Input: part model. Units: mm. Frame: model coordinates. Coordinates: 2 decimals unless noted, no trailing zeros. Write each loop counter-clockwise with the first axis right and the second up, starting at its lowest first coordinate (ties: lowest second). Pieces come first, ordered by that corner, then holes. Notation, with made-up numbers: M -18,60.5 L 35,60.5 A26 cw 35,81.5 Z; hole C 10.25,17.25 d9. An arc over 180 degrees is marked long. Answer as a JSON object with one key per item and string values. Group by question number.
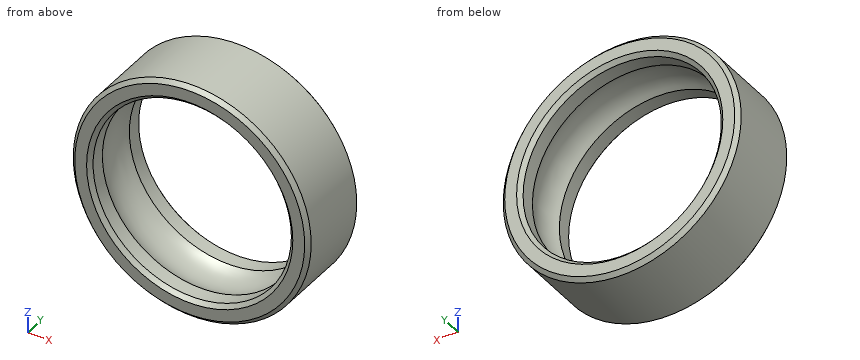
from build123d import *

# Parameters (mm, degrees)
SKETCH1_R           = 6
SKETCH1_R_2         = 5
BOSS_EXTRUDE1_DEPTH = 2
CHAMFER1_SIZE       = 0.2
SKETCH2_R           = 1.8


with BuildPart() as part:
    # Sketch1 → Boss-Extrude1 (new body, symmetric)
    with BuildSketch(Plane(origin=(0, 0, 0), x_dir=(1, 0, 0), z_dir=(0, 1, 0))):
        Circle(SKETCH1_R)
        Circle(SKETCH1_R_2, mode=Mode.SUBTRACT)
    extrude(amount=BOSS_EXTRUDE1_DEPTH, both=True)

    # Chamfer1
    chamfer1_edges = [part.edges().sort_by_distance(p)[0] for p in [
        (-6, -2, 0),
        (-6, 2, 0),
        (-5, -2, 0),
        (-5, 2, 0),
    ]]
    chamfer(chamfer1_edges, length=CHAMFER1_SIZE)

    # Cut-Sweep1: sweep along a path in Sketch3
    with BuildLine(Plane(origin=(0, 0, 0), x_dir=(1, 0, 0), z_dir=(0, 1, 0))) as cut_sweep1_path:
        CenterArc((0, 0), 3.542184236, 0, 360)
    # Sketch2 → Cut-Sweep1 (sweep, cut)
    with BuildSketch(Plane(origin=(0, 0, 0), x_dir=(0, 0, -1), z_dir=(1, 0, 0))):
        with Locations((-3.549093178, 0)):
            Circle(SKETCH2_R)
    sweep(path=cut_sweep1_path.line, mode=Mode.SUBTRACT)


solid = part.part
Q1. Section A-A, the plane x = 0. Return the cut outline in (y, z), and give its area (3 significant figures).
Q2. Line query: line 1 (X direction, y = 1.6, z = 0); line 2 (Z direction, x = -2, y = 0.75). Output: solid intervals per line, ascending. Write a range as from..to.
Q3. Pin query (flat end, axial travel): pin 1 Ø3 at (x, z) = (-0.5, -3.5) entering from -Y; pin 2 Ø1.5 at (y, z) = (-1.5, 1) entering from +X; pin 3 Ø1.5 at (x, z) = (3.5, -2.5) entering from -Y; pin 4 Ø3 at (x, z) = (-1.5, 2) entering from +Y. Return the tip coordinate at first contact, or that it passes through.
Q4. Section B-B, the plane z = 0. Return the cut outline in (x, y), and give its area (3 significant figures).
Q5. Section C-C, the plane y = -0.3. Return the cut outline in (x, z).
Q6. Section D-D, the plane y = 0.9. Return the cut outline in (x, z).
Filled in:
{
 "1": {"outline": "M -2,-5.8 L -1.8,-6 L 1.8,-6 L 2,-5.8 L 2,-5.2 L 1.8,-5 L 1.07,-5 A1.8 cw -1.07,-5 L -1.8,-5 L -2,-5.2 Z; M -2,5.2 L -1.8,5 L -1.07,5 A1.8 cw 1.07,5 L 1.8,5 L 2,5.2 L 2,5.8 L 1.8,6 L -1.8,6 L -2,5.8 Z", "area": "6.83 mm^2"},
 "2": {"line 1": "-6..-5, 5..6", "line 2": "-5.66..-4.78, 4.78..5.66"},
 "3": {"pin 1": "y = -1.84", "pin 2": "x = 5.99", "pin 3": "y = -1.85", "pin 4": "through"},
 "4": {"outline": "M -6,-1.8 L -5.8,-2 L -5.2,-2 L -5,-1.8 L -5,-1.07 A1.8 cw -5,1.07 L -5,1.8 L -5.2,2 L -5.8,2 L -6,1.8 Z; M 5,-1.8 L 5.2,-2 L 5.8,-2 L 6,-1.8 L 6,1.8 L 5.8,2 L 5.2,2 L 5,1.8 L 5,1.07 A1.8 cw 5,-1.07 Z", "area": "6.83 mm^2"},
 "5": {"outline": "C 0,0 d12; hole C 0,0 d10.65"},
 "6": {"outline": "C 0,0 d12; hole C 0,0 d10.22"}
}
